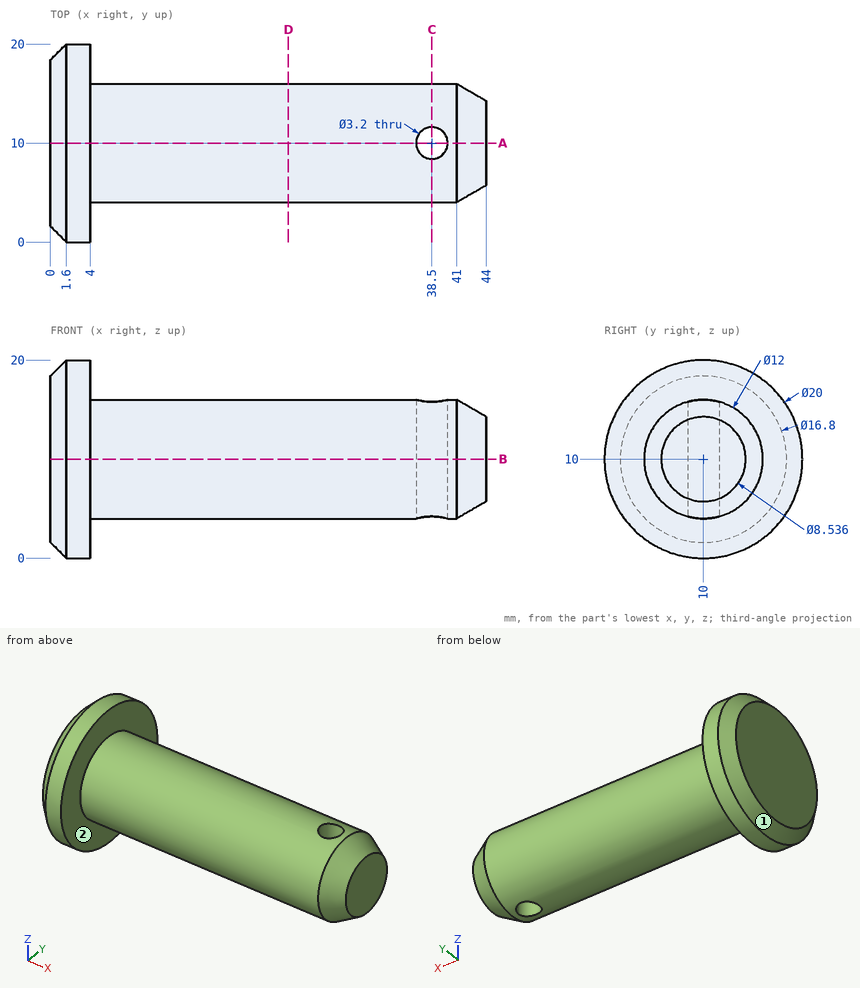
Input: dimensioned drawing with shaded views. Units: mm. Origin: part minimum x, y, z. A direction names the side the tool comes from. Round coordinates to 2 decimals unless told otherwise and drop trailing zeros. Loops run counter-clockwise (first coordinate to the right, second up) from the corner with the lowest first, then second, coordinate; pieces in that order, holes last. Notation, with made-up numbers: (33, 72) -> (42, 72) arc R27 ccw to (42, 101) -> close; hole circle Ø2 at (59, -0.75). An arc over 180 degrees is marked (long way). Use one line per item in the form item = value. Start each with the question number.
1) Access query for the marked faces 1 and 2. Directions: +Z, -Z, +X, -X, +Y, -Y. A direction counts if a zero-diameter tool reaches every point of the face in a straight line with its end or side. Return the directions, or none.
2) Section B-B on z = 10. Output: boundary loops of the cut face in (x, y), then the cut area to 3 significant figures.
3) Line query: L1, parallel to X at y = 10, z = 12; L2, parallel to X at y = 4.75, z = 7; L3, parallel to Y at x = 38.5, z = 8. Output: solid intervals per line, ascending.
4) Section D-D on x = 24. Output: boundary loops of the cut face in (y, z).
5) Section C-C on x = 38.5. Output: boundary loops of the cut face in (y, z).
6) Section A-A on y = 10. Output: boundary loops of the cut face in (x, z), then the cut area to 3 significant figures.
7) First-contact query: P1, Ø6, axis at x = 21, z = 6.5, coming from the +Y side; P2, Ø2, axis at x = 11, y = 7.5, coming from the -Z side; P3, Ø6, axis at x = 29, z = 14.5, coming from the -Y side. Flat tips, straight axial feed; report the tip coordinate or a pass-through.
Response:
q1.face_1 = -X
q1.face_2 = +X
q2.outline = (0, 1.6) -> (1.6, 0) -> (4, 0) -> (4, 4) -> (41, 4) -> (44, 5.73) -> (44, 14.27) -> (41, 16) -> (4, 16) -> (4, 20) -> (1.6, 20) -> (0, 18.4) -> close; hole circle Ø3.2 at (38.5, 10)
q2.area = 544 mm^2
q3.L1 = 0 to 36.9, 40.1 to 44
q3.L2 = 0 to 4
q3.L3 = 4.34 to 8.4, 11.6 to 15.66
q4.outline = circle Ø12 at (10, 10)
q5.outline = (8.4, 4.22) -> (8.4, 15.78) arc R6 ccw to start; (11.6, 4.22) arc R6 ccw to (11.6, 15.78) -> close
q6.outline = (0, 1.6) -> (1.6, 0) -> (4, 0) -> (4, 4) -> (36.9, 4) -> (36.9, 16) -> (4, 16) -> (4, 20) -> (1.6, 20) -> (0, 18.4) -> close; (40.1, 4) -> (41, 4) -> (44, 5.73) -> (44, 14.27) -> (41, 16) -> (40.1, 16) -> close
q6.area = 514 mm^2
q7.P1 = 15.98
q7.P2 = 4.19
q7.P3 = 4.19
